Design review of the part shown in the three views and the two pictorial views. Dimensions are in mm from the part's minimum x, y and z. Coordinates: 2 decimals unless noted, no trailing zeros. Loops run counter-clockwise (first coordinate to the right, second up) from the corner with the lowest first, then second, coordinate; pieces in that order, holes last. Notation, with made-up numbers: (-5, 39.5) -> (47, 39.5) arc R27 cw to (47, 65.5) -> close; hole circle Ø7 at (29, -24). An arc over 180 degrees is marked (long way). Use a Markdown table: item, result. Add a question column.
Q1. Take a section at B-B on x = 378. Write out the cut boundary in (y, z).
Q2. Take a section at A-A on y = 227. Write out the cut boundary in (x, z).
Q3. For probe 1 along Y at (x, z) = (255, 8); probe 2 along X at (y, z) = (177, 18.25), list the stretches that pass through material, from the lowest coordinate up.
Q4. Take a section at C-C on z = 12.25. Write out the cut boundary in (x, y), plus the area to 3 significant figures.
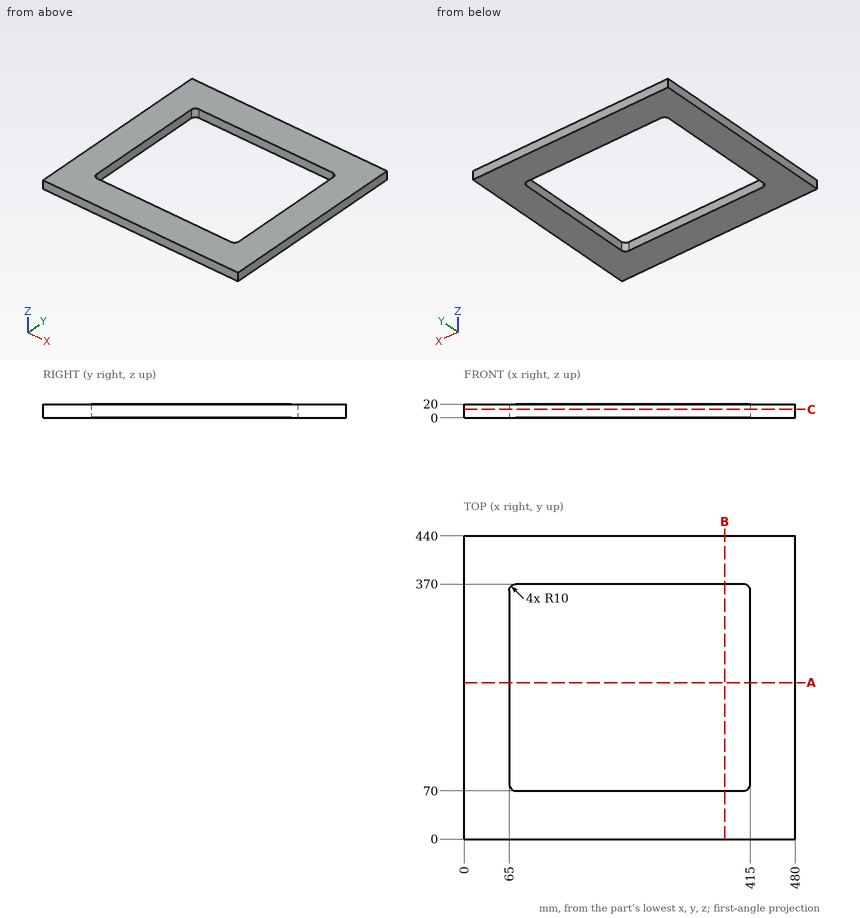
Answer list:
| question | item | result |
|---|---|---|
| 1 | outline | (0, 0) -> (70, 0) -> (70, 20) -> (0, 20) -> close; (370, 0) -> (440, 0) -> (440, 20) -> (370, 20) -> close |
| 2 | outline | (0, 0) -> (65, 0) -> (65, 20) -> (0, 20) -> close; (415, 0) -> (480, 0) -> (480, 20) -> (415, 20) -> close |
| 3 | probe 1 | 0 to 70, 370 to 440 |
| 3 | probe 2 | 0 to 65, 415 to 480 |
| 4 | outline | (0, 0) -> (480, 0) -> (480, 440) -> (0, 440) -> close; hole (65, 80) arc R10 ccw to (75, 70) -> (405, 70) arc R10 ccw to (415, 80) -> (415, 360) arc R10 ccw to (405, 370) -> (75, 370) arc R10 ccw to (65, 360) -> close |
| 4 | area | 106,000 mm² |
